```python
from build123d import *

# Parameters (mm, degrees)
SKETCH1_R           = 25.4
BASE_EXTRUDE_DEPTH  = 279.4
SKETCH2_R           = 12.7
BOSS_EXTRUDE1_DEPTH = 19.05


with BuildPart() as part:
    # Sketch1 → Base-Extrude (new, symmetric)
    with BuildSketch(Plane.XY):
        Circle(SKETCH1_R)
    extrude(amount=BASE_EXTRUDE_DEPTH, both=True)

    # Sketch2 → Boss-Extrude1 (add)
    with BuildSketch(Plane.XY.offset(279.4)):
        with Locations(Location((0, 0, 0), (0, 0, 180))):
            Circle(SKETCH2_R)
    boss_extrude1 = extrude(amount=BOSS_EXTRUDE1_DEPTH)

    # Mirror1: Boss-Extrude1 across plane
    add(boss_extrude1.mirror(Plane.XY))


solid = part.part
```
Can you work these out from the model? Positions are in its coordinate system, mm. A direction names the side the tool comes from. Give positions to 0.01 mm unless a question says otherwise; leave off trailing zeros. Order: outer loops, then holes, each group sorted by start corner. A loop starts at its lowest first (then second) coordinate and runs counter-clockwise, first axis right, second up. Notation, with made-up numbers: M -13.5,68 L 27.5,68 A30 ccw 27.5,95 Z; hole C 83,-23.75 d7. An arc over 180 degrees is marked long. Write item = value, one per line. Start each with the question number.
Q1. For faces 4 (the cylindrical face through (-5.86, 11.267, 288.792)), 5 (the flat face through (0, 0, 298.45)), 6 (the cylindrical face through (-5.86, 11.267, -288.792)), which set-ups out of +Z, -Z, +X, -X, +Y, -Y let a thin tool reach every point of the face, with its end or its side?
Q2. Suppose I cut it at C-C (z = 82). Write out the boundary of the cut face in (x, y), plus the area to 3 significant figures.
Q3. We'd pull the mould along Z, two halves only. Please class faces 1 (the flat face through (5, 12, -279.4)), 2 (the flat face through (5, 12, 279.4)), 3 (the cylindrical face through (-5.506, -24.796, 3.912)): pulls with the +Z half, pulls with the -Z half, needs draft (parallel to the pull), parting line crosses it, or undercut.
Q4. Suppose I cut it at A-A (y = 0). Write out the boundary of the cut face in (x, z), plus the area to 3 significant figures.
Q5. Suppose I cut it at B-B (x = -4.5). Write out the boundary of the cut face in (y, z).
Q6. Will these pins go through, and if not, where does the flat tip stop? pin 1 Ø1.5 at (y, z) = (-6.5, 197.5) entering from -X; pin 2 Ø6 at (y, z) = (-14, 236.5) entering from +X; pin 3 Ø2 at (x, z) = (15.5, 120.5) entering from -Y.
Q7. I need wall thicknesses on probe 1 along Z at (x, y) = (3, -14.5); probe 2 along X at (y, z) = (-2, -79.5); probe 3 along Y at (x, z) = (-1, 81). Which ranges of each line are inside material? Lowest first, please. Write a range as [from, to].
Check result:
q1.face_4 = +Z
q1.face_5 = +Z, +X, -X, +Y, -Y
q1.face_6 = -Z
q2.outline = C 0,0 d50.8
q2.area = 2,030 mm2
q3.face_1 = pulls with the -Z half
q3.face_2 = pulls with the +Z half
q3.face_3 = needs draft
q4.outline = M -25.4,-279.4 L -12.7,-279.4 L -12.7,-298.45 L 12.7,-298.45 L 12.7,-279.4 L 25.4,-279.4 L 25.4,279.4 L 12.7,279.4 L 12.7,298.45 L -12.7,298.45 L -12.7,279.4 L -25.4,279.4 Z
q4.area = 29,400 mm2
q5.outline = M -25,-279.4 L -11.88,-279.4 L -11.88,-298.45 L 11.88,-298.45 L 11.88,-279.4 L 25,-279.4 L 25,279.4 L 11.88,279.4 L 11.88,298.45 L -11.88,298.45 L -11.88,279.4 L -25,279.4 Z
q6.pin_1 = -24.74
q6.pin_2 = 22.89
q6.pin_3 = -20.85
q7.probe_1 = [-279.4, 279.4]
q7.probe_2 = [-25.32, 25.32]
q7.probe_3 = [-25.38, 25.38]
